```python
from build123d import *

# Parameters (mm, degrees)
SKETCH1_W           = 40
SKETCH1_H           = 150
BOSS_EXTRUDE1_DEPTH = 8
SKETCH2_W           = 10
SKETCH2_H           = 150
CUT_EXTRUDE1_DEPTH  = 5
SKETCH5_R           = 1.6
CUT_EXTRUDE2_DEPTH  = 35
SKETCH6_W           = 36
SKETCH6_H           = 14
CUT_EXTRUDE3_DEPTH  = 3
SKETCH7_R           = 1.6
CUT_EXTRUDE4_DEPTH  = 10
SKETCH8_R           = 1.6
CUT_EXTRUDE5_DEPTH  = 10
SKETCH9_R           = 1.6
CUT_EXTRUDE6_DEPTH  = 10


with BuildPart() as part:
    # Sketch1 → Boss-Extrude1 (new body)
    with BuildSketch(Plane.XY):
        with Locations((1.904761905, -44.285714286)):
            Rectangle(SKETCH1_W, SKETCH1_H)
    extrude(amount=BOSS_EXTRUDE1_DEPTH)

    # Sketch2 → Cut-Extrude1 (cut)
    with BuildSketch(Plane.XY):
        with Locations((-13.095238095, -44.285714286)):
            Rectangle(SKETCH2_W, SKETCH2_H)
    extrude(amount=CUT_EXTRUDE1_DEPTH, mode=Mode.SUBTRACT)

    # Sketch5 → Cut-Extrude2 (cut)
    with BuildSketch(Plane.XY.offset(8)):
        with Locations((10.404761905, 20.714285714)):
            Circle(SKETCH5_R)
        with Locations((-6.595238095, 20.714285714)):
            Circle(SKETCH5_R)
    extrude(amount=-CUT_EXTRUDE2_DEPTH, mode=Mode.SUBTRACT)

    # Sketch6 → Cut-Extrude3 (cut)
    with BuildSketch(Plane.XY.offset(8)):
        with Locations((1.904761905, -12.285714286)):
            Rectangle(SKETCH6_W, SKETCH6_H)
    extrude(amount=-CUT_EXTRUDE3_DEPTH, mode=Mode.SUBTRACT)

    # Sketch7 → Cut-Extrude4 (cut)
    with BuildSketch(Plane.XY.offset(8)):
        with Locations((-7.095238095, -44.285714286)):
            Circle(SKETCH7_R)
        with Locations((10.904761905, -44.285714286)):
            Circle(SKETCH7_R)
    extrude(amount=-CUT_EXTRUDE4_DEPTH, mode=Mode.SUBTRACT)

    # Sketch8 → Cut-Extrude5 (cut)
    with BuildSketch(Plane.XY.offset(8)):
        with Locations((-13.095238095, -89.285714286)):
            Circle(SKETCH8_R)
        with Locations((16.904761905, -89.285714286)):
            Circle(SKETCH8_R)
    extrude(amount=-CUT_EXTRUDE5_DEPTH, mode=Mode.SUBTRACT)

    # Sketch9 → Cut-Extrude6 (cut)
    with BuildSketch(Plane.XY.offset(8)):
        with Locations((-13.095238095, -99.285714286)):
            Circle(SKETCH9_R)
        with Locations((16.904761905, -99.285714286)):
            Circle(SKETCH9_R)
    extrude(amount=-CUT_EXTRUDE6_DEPTH, mode=Mode.SUBTRACT)


solid = part.part
```
Input: part model. Units: mm. Frame: model coordinates. A direction names the side the tool comes from. Coordinates: 2 decimals unless noted, no trailing zeros. Write each loop counter-clockwise with the first axis right and the second up, starting at its lowest first coordinate (ties: lowest second). Pieces come first, ordered by that corner, then holes. Notation, with made-up numbers: (-36, -1) - (14, -1) arc R22 ccw to (14, 16) - close; hole circle Ø5 at (10.25, 49.25). An arc over 180 degrees is marked (long way). Put each result on its own line as item: value. Start each with the question number.
1) Mould query, pull axis X, two halves, no side actions, for faces 1 (the face through (-13.44, -100.85, 6.52)), 2 (the face through (21.905, -45, 4)), 3 (the face through (7, -43, 0)). Classes: pulls with the +X half, pulls with the -X half, needs draft (parallel to the pull), parting line crosses it, or undercut.
2) Reachability of faces 4 (the face through (6, -12, 5)), 5 (the face through (-13, -43, 5)), 6 (the face through (-16.095, -12, 7)), 7 (the face through (6, 30.714, 4)) from +Z, -Z, +X, -X, +Y, -Y: full face, straight path, thin tool, end or side. Return the list, or none.
3) Contact query for flat-ended pins moving along their axis: pin 1 (3 mm diameter, centred on x = -13.1, y = -89.29, fed in from +Z); pin 2 (1.5 mm diameter, centred on y = -37.5, z = 2.5, fed in from -X). Output: stop coordinate, or through.
4) Cut plane C-C (z = 3.5). Return the cut outline in (x, y).
5) Cut plane A-A (y = -9.5). Return the cut outline in (x, z), plus the area to 3 significant figures.
6) Cut plane B-B (x = 0.5). Return the cut outline in (y, z).
7) Ray query, L1, parallel to Y at x = -13, z = 7.25; L2, parallel to Y at x = 10, z = 5.5; L3, parallel to Y at x = -10, z = 6. Return the intervals inside material, ascending.
8) Cut plane D-D (y = -84). Return the cut outline in (x, z).
Resolved:
1. face 1: undercut
1. face 2: pulls with the +X half
1. face 3: needs draft
2. face 4: +Z
2. face 5: -Z, -X, +Y, -Y
2. face 6: +Z, -Z
2. face 7: +Z, -Z, +X, -X, +Y
3. pin 1: passes through
3. pin 2: stops at x = -8.1
4. outline: (-8.1, -119.29) - (21.9, -119.29) - (21.9, 30.71) - (-8.1, 30.71) - (-8.1, 21.27) arc R1.6 cw (long way) to (-8.1, 20.16) - (-8.1, -43.04) arc R1.6 cw (long way) to (-8.1, -45.53) - close; hole circle Ø3.2 at (10.4, 20.71); hole circle Ø3.2 at (10.9, -44.29); hole circle Ø3.2 at (16.9, -99.29); hole circle Ø3.2 at (16.9, -89.29)
5. outline: (-18.1, 5) - (-16.1, 5) - (-16.1, 8) - (-18.1, 8) - close; (-8.1, 0) - (21.9, 0) - (21.9, 8) - (19.9, 8) - (19.9, 5) - (-8.1, 5) - close
5. area: 162 mm2
6. outline: (-119.29, 0) - (30.71, 0) - (30.71, 8) - (-5.29, 8) - (-5.29, 5) - (-19.29, 5) - (-19.29, 8) - (-119.29, 8) - close
7. L1: y = -119.29 to -100.88, -97.69 to -90.88, -87.69 to -19.29, -5.29 to 30.71
7. L2: y = -119.29 to -45.61, -42.97 to -19.29, -5.29 to 19.17, 22.26 to 30.71
7. L3: y = -119.29 to -19.29, -5.29 to 30.71
8. outline: (-18.1, 5) - (-8.1, 5) - (-8.1, 0) - (21.9, 0) - (21.9, 8) - (-18.1, 8) - close
